Can you work these out from the model? Positions are in its coordinate system, mm. Round coordinates to 2 decimals unless told otherwise and drop trailing zeros. Loops run counter-clockwise (first coordinate to the right, second up) from the corner with the lowest first, then second, coordinate; pieces in that order, holes last.
(1) I want a section at A-A on z = -19.5. Write out the boundary of the cut face in (x, y).
(2) Will these pins go through, and if not, where does the flat tip stop? pin 1 Ø1 at (y, z) = (21, -25) entering from -X; pin 2 Ø5 at (y, z) = (29.5, -27.5) entering from -X; pin 3 Ø6 at (y, z) = (35.5, -7) entering from -X.
(3) I want a section at C-C on z = -8.5. Write out the boundary of the cut face in (x, y).
(4) If I drill on line 1 along Z through (x, y) = (27, 28); line 2 along X through (y, z) = (18, -17.5); line 3 along Z through (x, y) = (15, 12), over which ranges is the centre line in solid material (lowest first)?
(5) I want a section at B-B on y = 20. Write out the boundary of the cut face in (x, z), plus the area to 3 significant figures.
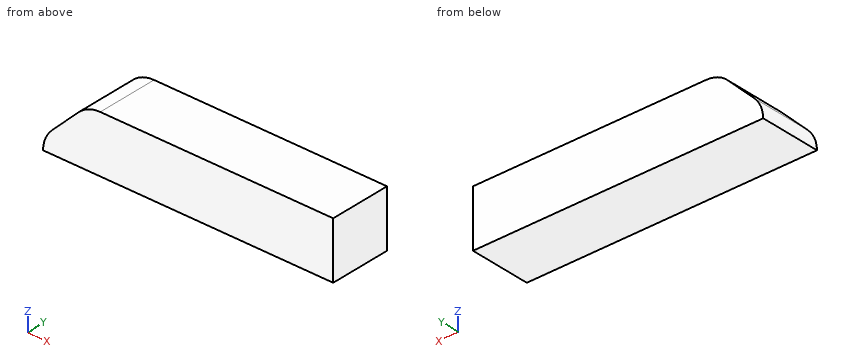
Solid Edge part; units mm, degrees
sketch "Sketch1" plane through (0, 0, 0) normal (0, -1, 0) x (1, 0, 0)
  line L0 (0, -37) -> (189, -37)
  line L1 (189, -37) -> (189, 0)
  line L2 (189, 0) -> (0, 0)
  line L3 (0, 0) -> (0, -37)
extrude "Protrusion1" add sketch "Sketch1" against normal blind 40
sketch "Sketch2" plane through (94.5, 0, -18.5) normal (0, -1, 0) x (1, 0, 0)
  line L0 (-65.5, 18.5) -> (-94.5, -10.5)
  line L1 (-94.5, -10.5) -> (-94.5, 18.5)
  line L2 (-94.5, 18.5) -> (-65.5, 18.5)
extrude "ExtrudedCutout_1" cut sketch "Sketch2" against normal blind 40
fillet "Round_1" radius 20 2 edges at (29, 20, 0) (0, 20, -29)
Filled sheet:
1. outline: (9.5, 0) - (189, 0) - (189, 40) - (9.5, 40) - close
2. pin 1: stops at x = 3.84
2. pin 2: stops at x = 1.37
2. pin 3: stops at x = 19
3. outline: (20.5, 0) - (189, 0) - (189, 40) - (20.5, 40) - close
4. line 1: z = -37 to -2.85
4. line 2: x = 11.5 to 189
4. line 3: z = -37 to -14
5. outline: (0, -37) - (189, -37) - (189, 0) - (37.28, 0) arc R20 ccw to (23.14, -5.86) - (5.86, -23.14) arc R20 ccw to start
5. area: 6,560 mm2
